Geometry: see drawing. Coordinates: mm, zero at the bounding-box minimum. A direction names the side the tool comes from. Coordinates: 2 decimals unless noted, no trailing zeros. Loops run counter-clockwise (first coordinate to the right, second up) from the corner with the lowest first, then second, coordinate; pieces in that order, holes last. Notation, with made-up numbers: M 34.5,-11 L 44.5,-11 A20 cw 44.5,-5 Z; hole C 12,-15 d2. An arc over 180 degrees is marked long. One line per question, with ' | ' between items. Start each with the question number.
1. Section query D-D, the plane y = 4.5. Output: boundary loops of the cut face in (x, z), and give its area (3 significant figures).
2. Ray query, probe 1 along X at (y, z) = (12.25, 7); probe 2 along Z at (x, y) = (4, 4); probe 3 along Y at (x, z) = (7.5, 14). Return the intervals inside material, ascending.
3. Access query for the marked faces 5 and 6. Directions: +Z, -Z, +X, -X, +Y, -Y. A direction counts if a zero-diameter tool reaches every point of the face in a straight line with its end or side. Return the directions, or none.
4. Section query C-C, the plane z = 14. Output: boundary loops of the cut face in (x, y), and give its area (3 significant figures).
5. Section query A-A, the plane x = 12. Output: boundary loops of the cut face in (y, z), and give its area (3 significant figures).
6. Section query B-B, the plane z = 22.75. Output: boundary loops of the cut face in (x, y).
7. Mould query, pull axis Z, two halves, no side actions, for the marked faces 1, 2, 3 and 4. Classes: pulls with the +Z half, pulls with the -Z half, needs draft (parallel to the pull), parting line crosses it, or undercut.
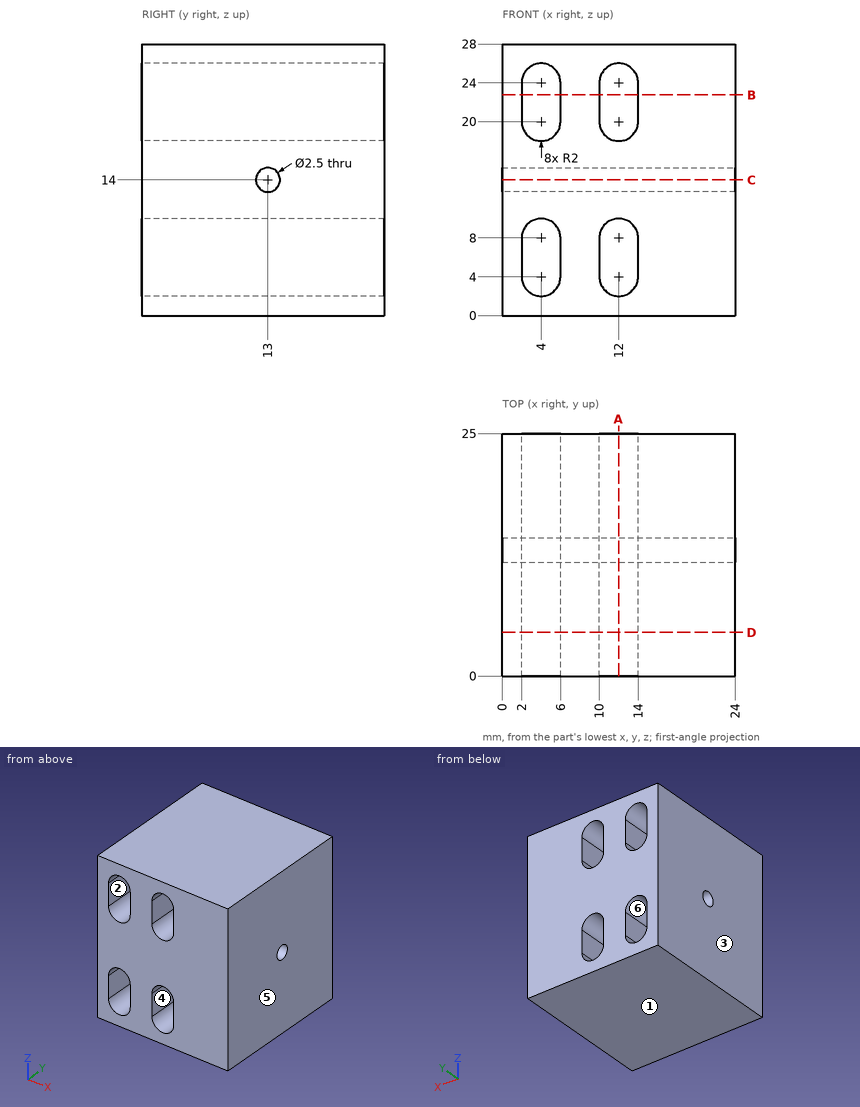
Taken from the geometry:
1) outline: M 0,0 L 24,0 L 24,28 L 0,28 Z; hole M 2,4 A2 ccw 6,4 L 6,8 A2 ccw 2,8 Z; hole M 2,20 A2 ccw 6,20 L 6,24 A2 ccw 2,24 Z; hole M 10,4 A2 ccw 14,4 L 14,8 A2 ccw 10,8 Z; hole M 10,20 A2 ccw 14,20 L 14,24 A2 ccw 10,24 Z | area: 558 mm^2
2) probe 1: 0 to 2, 6 to 10, 14 to 24 | probe 2: 0 to 2, 10 to 18, 26 to 28 | probe 3: 0 to 11.75, 14.25 to 25
3) face 5: +Z, -Z, +X, +Y, -Y | face 6: +Y, -Y
4) outline: M 0,0 L 24,0 L 24,11.75 L 0,11.75 Z; M 0,14.25 L 24,14.25 L 24,25 L 0,25 Z | area: 540 mm^2
5) outline: M 0,0 L 25,0 L 25,2 L 0,2 Z; M 0,10 L 25,10 L 25,18 L 0,18 Z; M 0,26 L 25,26 L 25,28 L 0,28 Z; hole C 13,14 d2.5 | area: 295 mm^2
6) outline: M 0,0 L 2,0 L 2,25 L 0,25 Z; M 6,0 L 10,0 L 10,25 L 6,25 Z; M 14,0 L 24,0 L 24,25 L 14,25 Z
7) face 1: pulls with the -Z half | face 2: undercut | face 3: needs draft | face 4: undercut
